Check sheet for the drawn part. Datum: minimum x, y, z corner. Units: mm. Coordinates: 2 decimals unless noted, no trailing zeros. Loops run counter-clockwise (first coordinate to the right, second up) from the corner with the lowest first, then second, coordinate; pieces in that order, holes last. Notation, with made-up numbers: M 14,21.25 L 46,21.25 A18 ccw 46,43.25 Z; hole C 29,-20.5 d8. An arc over 180 degrees is marked long. Use CSV: the item, a comma, the result in double quotes. Start each with the question number.
(1) Section check B-B on x = 13.25. Record the cut outline in (y, z), and give its area (3 significant figures).
(2) Scan lines: line 1 (X direction, y = 54.5, z = 1); line 2 (Y direction, x = 23, z = 2.35); line 3 (Y direction, x = 27.5, z = 2.15). Record each from-to range of solid material in increasing order.
(3) Go/stop test with flat-tipped pins: pin 1 Ø1.5 at (y, z) = (55.5, 2) entering from -X; pin 2 Ø0.9 at (x, z) = (21.5, 1) entering from +Y. Record where each tip stops, or that it passes through.
(4) Section check D-D on x = 23. Record the cut outline in (y, z), and give its area (3 significant figures).
(5) Section check C-C on y = 8. Record the cut outline in (x, z).
(6) Section check A-A on z = 0.65. Record the cut outline in (x, y), and give its area (3 significant figures).
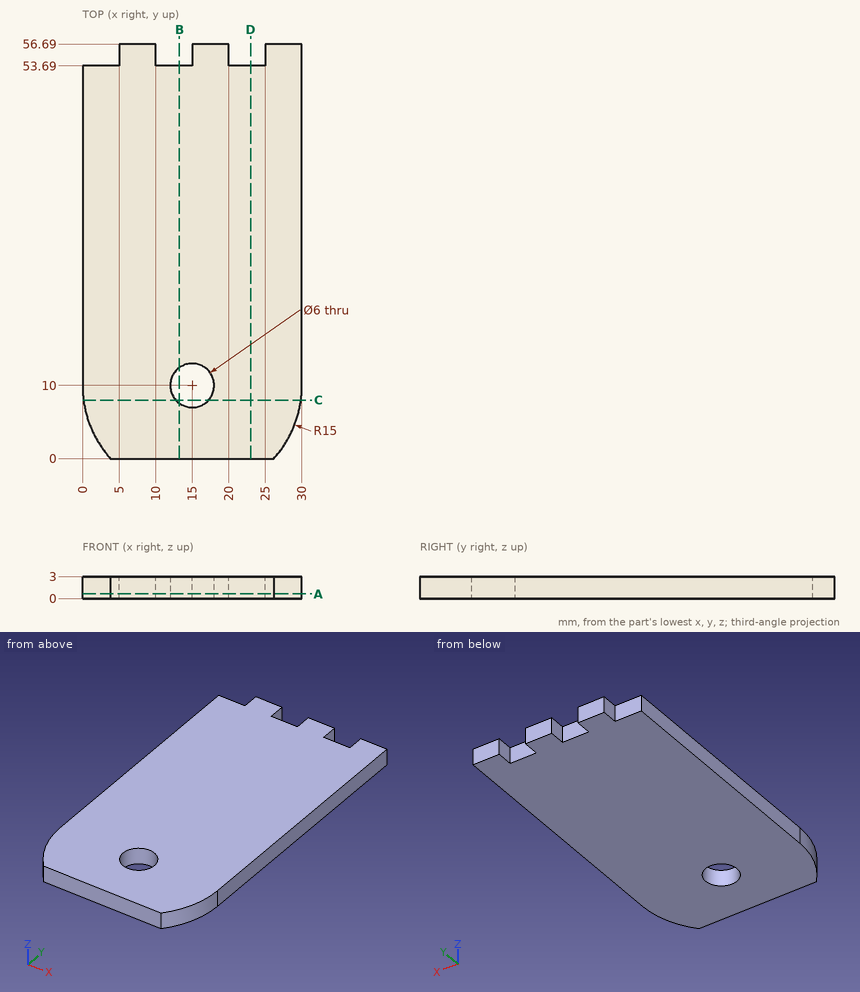
Outcome:
1,outline,"M 0,0 L 7.56,0 L 7.56,3 L 0,3 Z; M 12.44,0 L 53.69,0 L 53.69,3 L 12.44,3 Z"
1,area,"146 mm²"
2,line 1,"x = 5 to 10, 15 to 20, 25 to 30"
2,line 2,"y = 0 to 53.69"
2,line 3,"y = 1.71 to 56.69"
3,pin 1,"stops at x = 5"
3,pin 2,"stops at y = 53.69"
4,outline,"M 0,0 L 53.69,0 L 53.69,3 L 0,3 Z"
4,area,"161 mm²"
5,outline,"M 0.13,0 L 12.76,0 L 12.76,3 L 0.13,3 Z; M 17.24,0 L 29.87,0 L 29.87,3 L 17.24,3 Z"
6,outline,"M 0,10 A15 ccw 3.82,0 L 26.18,0 A15 ccw 30,10 L 30,56.69 L 25,56.69 L 25,53.69 L 20,53.69 L 20,56.69 L 15,56.69 L 15,53.69 L 10,53.69 L 10,56.69 L 5,56.69 L 5,53.69 L 0,53.69 Z; hole C 15,10 d6"
6,area,"1,600 mm²"
